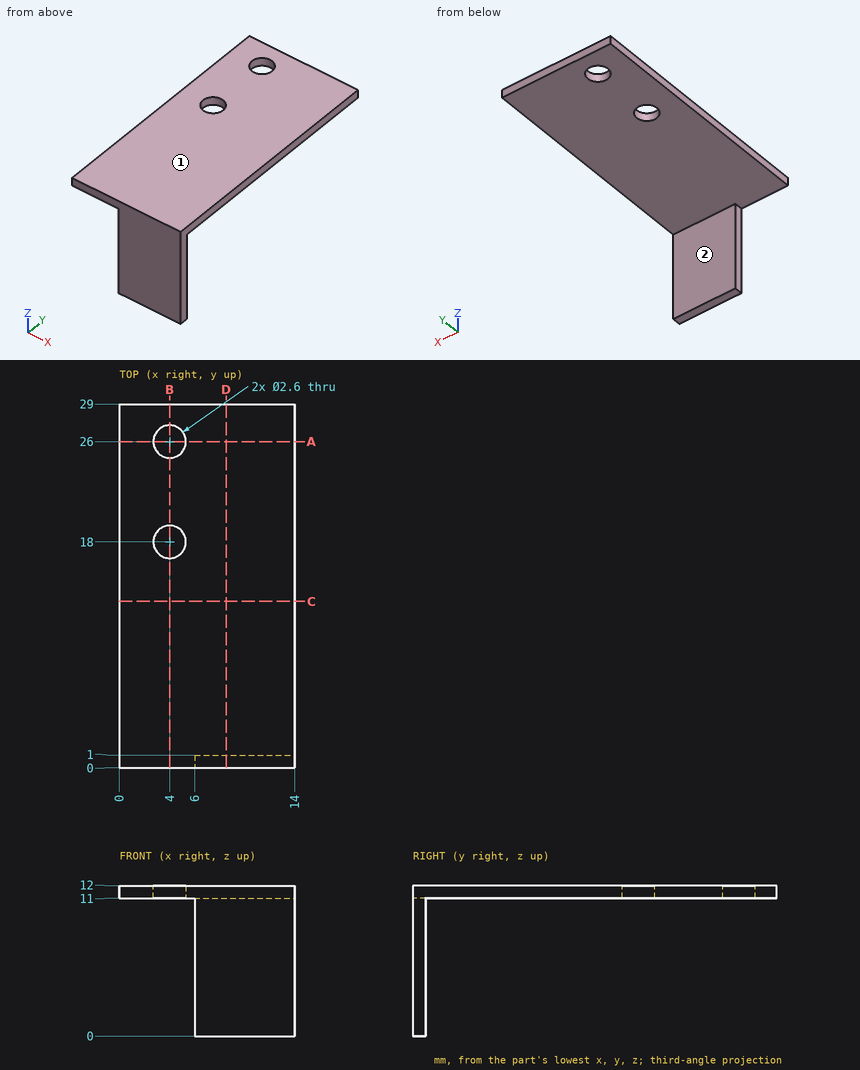
Here's the drawing with two shaded views (mm, measured from the low corner). I have some questions. A direction names the side the tool comes from. Give positions to 0.01 mm unless a question says otherwise; leave off trailing zeros. Order: outer loops, then holes, each group sorted by start corner. A loop starts at its lowest first (then second) coordinate and runs counter-clockwise, first axis right, second up. Notation, with made-up numbers: M -9.75,13.25 L 27.25,13.25 A14 ccw 27.25,32.25 Z; hole C 11,-12 d2. An arc over 180 degrees is marked long. Answer as a JSON object with one key per item and string values. Group by question number.
1) Suppose I cut it at A-A, the plane y = 26. Write out the boundary of the cut face in (x, z), plus the area to 3 significant figures.
2) Suppose I cut it at B-B, the plane x = 4. Write out the boundary of the cut face in (y, z), plus the area to 3 significant figures.
3) Suppose I cut it at C-C, the plane y = 13.25. Write out the boundary of the cut face in (x, z), plus the area to 3 significant figures.
4) On a 3-axis mill with a long thin cutter (end or side, diameter ignored), from which of +Z, -Z, +X, -X, +Y, -Y can I reach the whole of each face in a straight line? I mean the marked faces 1 and 2. Say none if no direction works.
5) Please list where these lines run through material, in increasing order: L1, parallel to Y at x = 4, z = 11.6; L2, parallel to Z at x = 6.75, y = 7.5; L3, parallel to Y at x = 6.75, z = 3.5. Write a range as [from, to].
6) Suppose I cut it at D-D, the plane x = 8.5. Write out the boundary of the cut face in (y, z).
7) I'm going to push flat-ended pins straight in: pin 1 Ø4 at (x, y) = (5, 13) entering from -Z; pin 2 Ø5 at (x, z) = (7, 8) entering from +Y; pin 3 Ø1.5 at (y, z) = (10, 10) entering from -X; pin 4 Ø1.1 at (y, z) = (0.5, 7.5) entering from -X. Where does each tip first touch, or does it pass through?
Results found:
{
 "1": {"outline": "M 0,11 L 2.7,11 L 2.7,12 L 0,12 Z; M 5.3,11 L 14,11 L 14,12 L 5.3,12 Z", "area": "11.4 mm²"},
 "2": {"outline": "M 0,11 L 16.7,11 L 16.7,12 L 0,12 Z; M 19.3,11 L 24.7,11 L 24.7,12 L 19.3,12 Z; M 27.3,11 L 29,11 L 29,12 L 27.3,12 Z", "area": "23.8 mm²"},
 "3": {"outline": "M 0,11 L 14,11 L 14,12 L 0,12 Z", "area": "14.0 mm²"},
 "4": {"face 1": "+Z, +X, -X, +Y, -Y", "face 2": "-Z, +X, -X, +Y"},
 "5": {"L1": "[0, 16.7], [19.3, 24.7], [27.3, 29]", "L2": "[11, 12]", "L3": "[0, 1]"},
 "6": {"outline": "M 0,0 L 1,0 L 1,11 L 29,11 L 29,12 L 0,12 Z"},
 "7": {"pin 1": "z = 11", "pin 2": "y = 1", "pin 3": "through", "pin 4": "x = 6"}
}
